Work out the finished part from the listing and answer in its coordinate system (mm). Face numbers are marked on the shaded views. A direction names the side the tool comes from. Coordinates: 2 decimals unless noted, no trailing zeros. Order: outer loops, then holes, each group sorted by start corner. A loop starts at its lowest first (then second) coordinate and runs counter-clockwise, first axis right, second up.
1. Find the intervals of material crossed by probe 1 along Z at (x, y) = (11, -41.5); probe 2 along X at (y, z) = (-4.5, -23); probe 3 along Y at (x, z) = (-50, -12), in increasing order.
2. Determine the mould class of the marked faces 5, 6 and 7 for opening direction X: +X half, -X half, draft (parallel to the pull), parting line (faces both ways), or undercut.
3. A tool of negligible diameter and unlimited length cuts with its end or side. For the marked faces 1, 2, 3 and 4, from which of +Z, -Z, +X, -X, +Y, -Y can it reach the whole face along a straight path? Write none if from no direction.
4. The part is cut by section D-D, the plane y = -61.5. Give the vertices of the cut face in (x, z), then the cut area to 3 significant figures.
5. The part is cut by section C-C, the plane x = -46.5. Give the vertices of the cut face in (y, z).
6. The part is cut by section A-A, the plane z = -23.5. Give the vertices of the cut face in (x, y).
7. The part is cut by section B-B, the plane y = -20. Give the vertices of the cut face in (x, z).
8. Flat-ended cylindrical pins translate along their axes: pin 1 Ø6 at (x, y) = (20.5, -62.5) entering from +Z; pin 2 Ø12.5 at (x, z) = (-40, -16.5) entering from -Y; pin 3 Ø12.5 at (x, z) = (48.5, -18) entering from -Y. Find the tip coordinate at first contact, or state that the pin passes through.
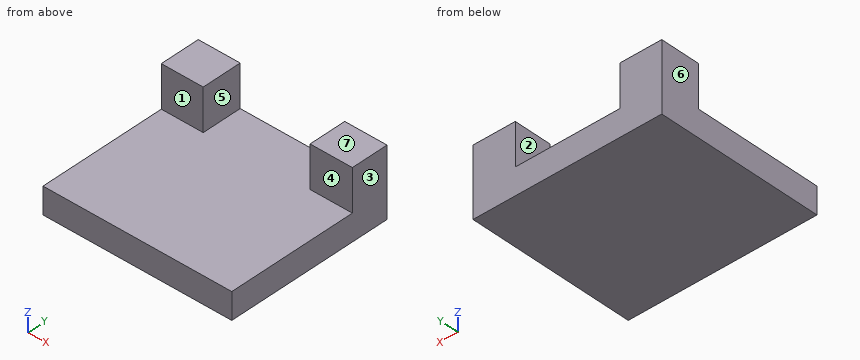
```python
from build123d import *

# Parameters (mm, degrees)
F0_W     = 114.5210824907
F0_H     = 16.0948559642
F1_DEPTH = 101.6
F2_W     = 25.6531313062
F2_H     = 22.6550512016
F3_DEPTH = 25.4
F4_W     = 25.4432931542
F4_H     = 15.3012713417
F5_DEPTH = 25.4
F6_DEPTH = 8.89


with BuildPart() as f1:
    # F0 (on Front) → F1 (new body)
    with BuildSketch(Plane.XZ):
        with Locations((0.928549096, -39.4633449614)):
            Rectangle(F0_W, F0_H)
    extrude(amount=F1_DEPTH)

    # F2 (on face) → F3 (join)
    with BuildSketch(Plane.XY.offset(-31.4159169793)):
        with Locations((45.3625246882, -11.3275256008)):
            Rectangle(F2_W, F2_H)
    extrude(amount=F3_DEPTH)

    # F4 (on face) → F5 (join)
    with BuildSketch(Plane.XY.offset(-31.4159169793)):
        with Locations((-43.6103455722, -7.6506356709)):
            Rectangle(F4_W, F4_H)
    extrude(amount=F5_DEPTH)

    # F6 (add): a face of the model
    f6_faces = [f1.faces().sort_by_distance(p)[0] for p in [
        (-43.6103455722, -15.3012713417, -18.7159169793),
    ]]
    extrude(f6_faces, amount=F6_DEPTH)


solid = f1.part
```
Geometry says:
1. probe 1: z = -47.51 to -31.42
1. probe 2: x = -56.33 to -30.89, 32.54 to 58.19
1. probe 3: y = -24.19 to 0
2. face 5: undercut
2. face 6: -X half
2. face 7: draft
3. face 1: +Z, +X, -X, -Y
3. face 2: +Z, +Y, -Y
3. face 3: +Z, -Z, +X, +Y, -Y
3. face 4: +Z, +X, -Y
4. outline: (-56.33, -47.51) - (58.19, -47.51) - (58.19, -31.42) - (-56.33, -31.42) - close
4. area: 1,840 mm2
5. outline: (-101.6, -47.51) - (0, -47.51) - (0, -6.02) - (-24.19, -6.02) - (-24.19, -31.42) - (-101.6, -31.42) - close
6. outline: (-56.33, -24.19) - (-30.89, -24.19) - (-30.89, 0) - (-56.33, 0) - close; (32.54, -22.66) - (58.19, -22.66) - (58.19, 0) - (32.54, 0) - close
7. outline: (-56.33, -47.51) - (58.19, -47.51) - (58.19, -6.02) - (32.54, -6.02) - (32.54, -31.42) - (-30.89, -31.42) - (-30.89, -6.02) - (-56.33, -6.02) - close
8. pin 1: stops at z = -31.42
8. pin 2: stops at y = -24.19
8. pin 3: stops at y = -22.66
